The model under review builds one solid part; all positions refer to its coordinate system, in mm. A direction names the side the tool comes from. Coordinates: 2 decimals unless noted, no trailing zeros. Loops run counter-clockwise (first coordinate to the right, second up) from the corner with the lowest first, then second, coordinate; pieces in that order, holes last. Notation, with made-up numbers: (41, 17.25) - (56, 17.25) arc R29 ccw to (56, 38.25) - close; hole circle Ø5 at (41, 71.5). An arc over 180 degrees is marked (long way). Use a Markdown table: item, result. Add a question column.
1) For faces 4 (the flat face through (-505.46, 3, 250)), 5 (the flat face through (-7, -254, 250)), list the 3-axis set-ups (+Z, -Z, +X, -X, +Y, -Y) from which the entire face can be reached by the end or side of a thin tool; tool diameter is ignored.
2) Clearance check with flat-ended pins moving along their axes: pin 1 (5 mm diameter, centred on y = 213.51, z = 220, fed in from +X); pin 2 (0.8 mm diameter, centred on y = -252.5, z = 410, fed in from +X); pin 3 (5.5 mm diameter, centred on x = 420, z = 468, fed in from +Y). State where each tip first meets the part, or that it passes through.
3) To check wall thickness, follow L1, parallel to Y at x = 506.85, z = 220; L2, parallel to Y at x = 506.6, z = 220; L3, parallel to X at y = 252.6, z = 468. State the ranges of each line that lie inside material, in increasing order. Write a range as [from, to].
4) Add section A-A, the plane y = 98. Give the boundary of the cut face in (x, z).
5) Add section C-C, the plane z = 162. Give the boundary of the cut face in (x, y).
6) Add section B-B, the plane x = -180. Give the boundary of the cut face in (y, z).
7) The part is to be moulded in two halves that separate along Y. For faces 1 (the flat face through (505.46, -3, 250)), 2 (the flat face through (7, 254, 250)), 3 (the flat face through (-508, 3, 250)), say which applies: pulls with the +Y half, pulls with the -Y half, needs draft (parallel to the pull), parting line crosses it, or undercut.
```python
from build123d import *

# Parameters (mm, degrees)
F1_DEPTH  = 508
F2_T      = -2.54
F4_DEPTH  = 381
F6_DEPTH  = 635
F7_R      = 3.5
F8_DEPTH  = 254.001
F10_DEPTH = 254.001
F11_R     = 3
F12_DEPTH = 381
F13_R     = 3
F14_DEPTH = 1270


with BuildPart() as f1:
    # F0 (on Top) → F1 (new body)
    with BuildSketch(Plane.XY):
        with BuildLine():
            ThreePointArc((508, 247.65), (506.140128, 252.140128), (501.65, 254))
            Line((501.65, 254), (-501.65, 254))
            ThreePointArc((-501.65, 254), (-506.140128, 252.140128), (-508, 247.65))
            Line((-508, 247.65), (-508, -247.65))
            ThreePointArc((-508, -247.65), (-506.140128, -252.140128), (-501.65, -254))
            Line((-501.65, -254), (501.65, -254))
            ThreePointArc((501.65, -254), (506.140128, -252.140128), (508, -247.65))
            Line((508, -247.65), (508, 247.65))
        make_face()
    extrude(amount=F1_DEPTH)

    # F2
    f2_openings = [f1.faces().sort_by_distance(p)[0] for p in [
        (0, 0, 508),
        (0, 0, 0),
    ]]
    offset(amount=F2_T, openings=f2_openings)

    # F3 (on Front) → F4 (cut, symmetric)
    with BuildSketch(Plane.XZ):
        with BuildLine():
            ThreePointArc((431.8, 0), (0, 62.451246), (-431.8, 0))
            Line((-431.8, 0), (431.8, 0))
        make_face()
    extrude(amount=F4_DEPTH, both=True, mode=Mode.SUBTRACT)

    # F5 (on Right) → F6 (cut, symmetric)
    with BuildSketch(Plane.YZ):
        with BuildLine():
            Line((-177.8, 0), (177.8, 0))
            ThreePointArc((177.8, 0), (0, 35.988652), (-177.8, 0))
        make_face()
    extrude(amount=F6_DEPTH, both=True, mode=Mode.SUBTRACT)

    # F7 (on Front) → F8 (cut, through all)
    with BuildSketch(Plane.XZ):
        with Locations((420, 468)):
            Circle(F7_R)
        with Locations((140, 468)):
            Circle(F7_R)
        with Locations((-140, 468)):
            Circle(F7_R)
        with Locations((-420, 468)):
            Circle(F7_R)
    extrude(amount=-F8_DEPTH, mode=Mode.SUBTRACT)

    # F9 (on Front) → F10 (cut, through all)
    with BuildSketch(Plane.XZ):
        with BuildLine():
            Line((-9, 416.674676), (-9, 399.325324))
            ThreePointArc((-9, 399.325324), (0, 395.5), (9, 399.325324))
            Line((9, 399.325324), (9, 416.674676))
            ThreePointArc((9, 416.674676), (0, 420.5), (-9, 416.674676))
        make_face()
    extrude(amount=F10_DEPTH, mode=Mode.SUBTRACT)

    # F11 (on Front) → F12 (cut, symmetric)
    with BuildSketch(Plane.XZ):
        with Locations((-467.5124, 220)):
            Circle(F11_R)
        with Locations((-467.5124, 80)):
            Circle(F11_R)
        with Locations((467.5124, 220)):
            Circle(F11_R)
        with Locations((467.5124, 80)):
            Circle(F11_R)
    extrude(amount=F12_DEPTH, both=True, mode=Mode.SUBTRACT)

    # F13 (on Right) → F14 (cut, symmetric)
    with BuildSketch(Plane.YZ):
        with Locations((213.5124, 220)):
            Circle(F13_R)
        with Locations((213.5124, 80)):
            Circle(F13_R)
        with Locations((-213.5124, 220)):
            Circle(F13_R)
        with Locations((-213.5124, 80)):
            Circle(F13_R)
    extrude(amount=F14_DEPTH, both=True, mode=Mode.SUBTRACT)


solid = f1.part
```
From the geometry:
| question | item | result |
|---|---|---|
| 1 | face 4 | +Z, -Z |
| 1 | face 5 | +Z, -Z, +X, -X, -Y |
| 2 | pin 1 | passes through |
| 2 | pin 2 | stops at x = 506.18 |
| 2 | pin 3 | stops at y = -251.46 |
| 3 | L1 | y = [-251.29, -216.51], [-210.51, 210.51], [216.51, 251.29] |
| 3 | L2 | y = [-251.63, -216.51], [-210.51, 210.51], [216.51, 251.63] |
| 3 | L3 | x = [-505.63, -423.5], [-416.5, -143.5], [-136.5, 136.5], [143.5, 416.5], [423.5, 505.63] |
| 4 | outline | (-508, 25.36) - (-505.46, 25.36) - (-505.46, 508) - (-508, 508) - close; (505.46, 25.36) - (508, 25.36) - (508, 508) - (505.46, 508) - close |
| 5 | outline | (-508, -247.65) arc R6.35 ccw to (-501.65, -254) - (501.65, -254) arc R6.35 ccw to (508, -247.65) - (508, 247.65) arc R6.35 ccw to (501.65, 254) - (-501.65, 254) arc R6.35 ccw to (-508, 247.65) - close; hole (-505.46, -247.65) arc R3.81 ccw to (-501.65, -251.46) - (501.65, -251.46) arc R3.81 ccw to (505.46, -247.65) - (505.46, 247.65) arc R3.81 ccw to (501.65, 251.46) - (-501.65, 251.46) arc R3.81 ccw to (-505.46, 247.65) - close |
| 6 | outline | (-254, 51.78) - (-251.46, 51.78) - (-251.46, 508) - (-254, 508) - close; (251.46, 51.78) - (254, 51.78) - (254, 508) - (251.46, 508) - close |
| 7 | face 1 | undercut |
| 7 | face 2 | pulls with the +Y half |
| 7 | face 3 | needs draft |
